Verification items for the finished model (mm, model axes). Round coordinates to 2 decimals unless told otherwise and drop trailing zeros. Loops run counter-clockwise (first coordinate to the right, second up) from the corner with the lowest first, then second, coordinate; pieces in that order, holes last. Notation, with made-up numbers: (-39.75, 39) - (-25.75, 39) arc R34 ccw to (-25.75, 69) - close; hole circle Ø8 at (49.5, 82). An arc over 180 degrees is marked (long way). Use a Markdown table: item, result. Add a question column.
```python
from build123d import *

# Parameters (mm, degrees)
F0_R      = 12
F1_DEPTH  = 2
F3_DEPTH  = 2
F4_R      = 1.5
F5_DEPTH  = 25
F6_R      = 6.35
F7_DEPTH  = 25
F8_R      = 1.5
F9_DEPTH  = 25
F10_R     = 1.5
F11_DEPTH = 25
F12_SIZE  = 1.86


with BuildPart() as f1:
    # F0 (on Front) → F1 (new body)
    with BuildSketch(Plane.XZ):
        with BuildLine():
            ThreePointArc((64.5, -22.5), (87, 0), (64.5, 22.5))
            Line((64.5, 22.5), (-64.5, 22.5))
            ThreePointArc((-64.5, 22.5), (-87, 0), (-64.5, -22.5))
            Line((-64.5, -22.5), (64.5, -22.5))
        make_face()
        with Locations((-64.5, 0)):
            Circle(F0_R, mode=Mode.SUBTRACT)
        with Locations((64.5, 0)):
            Circle(F0_R, mode=Mode.SUBTRACT)
    extrude(amount=F1_DEPTH)

    # F2 (on face) → F3 (join)
    with BuildSketch(Plane.XZ.offset(2)):
        Polygon((-87, -22.5), (-64.5, -22.5), (-64.5, -17.4313578755), (-70.5482587218, -14.7617282346), (-78.2682448626, -9.4630774111), (-80.8771923184, 0), (-87, 0), align=None)
    extrude(amount=-F3_DEPTH)

    # F4 (on face) → F5 (cut)
    with BuildSketch(Plane.XZ.offset(2)):
        with Locations((-53.5, 16)):
            Circle(F4_R)
        with Locations((-53.5, -16)):
            Circle(F4_R)
        with Locations((53.5, 16)):
            Circle(F4_R)
        with Locations((53.5, -16)):
            Circle(F4_R)
    extrude(amount=-F5_DEPTH, mode=Mode.SUBTRACT)

    # F6 (on face) → F7 (cut)
    with BuildSketch(Plane.XZ.offset(2)):
        Circle(F6_R)
    extrude(amount=-F7_DEPTH, mode=Mode.SUBTRACT)

    # F8 (on face) → F9 (cut)
    with BuildSketch(Plane.XZ.offset(2)):
        with Locations((-11.35, 4)):
            Circle(F8_R)
        with Locations((-11.35, -4)):
            Circle(F8_R)
        with Locations((11.35, 4)):
            Circle(F8_R)
        with Locations((11.35, -4)):
            Circle(F8_R)
    extrude(amount=-F9_DEPTH, mode=Mode.SUBTRACT)

    # F10 (on face) → F11 (cut)
    with BuildSketch(Plane.XZ.offset(2)):
        with Locations((0, -12.5)):
            Circle(F10_R)
        with Locations((31.499365073, -12.7)):
            Circle(F10_R)
        with Locations((-31.5, -12.5)):
            Circle(F10_R)
        with Locations((-37.5, -3.5)):
            Circle(F10_R)
    extrude(amount=-F11_DEPTH, mode=Mode.SUBTRACT)

    # F12
    f12_edges = [f1.edges().sort_by_distance(p)[0] for p in [
        (-55, 0, -16),
        (-33, 0, -12.5),
        (-55, 0, 16),
        (-12.85, 0, -4),
        (-12.85, 0, 4),
        (-1.5, 0, -12.5),
        (9.85, 0, -4),
        (9.85, 0, 4),
        (29.999365, 0, -12.7),
        (52, 0, -16),
        (52, 0, 16),
        (-39, 0, -3.5),
    ]]
    chamfer(f12_edges, length=F12_SIZE)


solid = f1.part
```
Q1. Thickness scan on line 1 along Z through (x, y) = (11.35, -1.85); line 2 along Z through (x, y) = (0, -1.85); line 3 along Z through (x, y) = (-64.5, -0.45). Record the ranges inside material, lowest first.
Q2. Release check for a two-part mould opening along Z. For faces 1 (the face through (-80.234, -0.986, 16.084)), 2 (the face through (-76.49, -0.99, 0.53)), 3 (the face through (-1, 0, 10)), 4 (the face through (87, -1, 0)) record: +Z half, -Z half, draft (parallel to the pull), parting line (faces both ways), or undercut.
Q3. Go/stop test with flat-tipped pins: pin 1 Ø3.5 at (x, z) = (-11.35, 4) entering from -Y; pin 2 Ø2.5 at (x, z) = (31.5, -12.7) entering from -Y; pin 3 Ø5 at (x, z) = (53.5, -16) entering from +Y; pin 4 Ø1 at (y, z) = (-1.5, 15) entering from -X. Record where each tip stops, or that it passes through.
Q4. Section check C-C on x = -63. Record the cut outline in (y, z).
Q5. Section check B-B on y = -0.7. State how many separate pieces and enclosed holes the cut face has, plus the area to 3 significant figures.
Q6. Section check A-A on x = 11.35. Record the cut outline in (y, z), plus the area to 3 significant figures.
Determined:
| question | item | result |
|---|---|---|
| 1 | line 1 | z = -22.5 to -5.51, -2.49 to 2.49, 5.51 to 22.5 |
| 1 | line 2 | z = -22.5 to -14.01, -10.99 to -6.35, 6.35 to 22.5 |
| 1 | line 3 | z = -22.5 to -12, 12 to 22.5 |
| 2 | face 1 | +Z half |
| 2 | face 2 | undercut |
| 2 | face 3 | draft |
| 2 | face 4 | parting line |
| 3 | pin 1 | stops at y = -2 |
| 3 | pin 2 | passes through |
| 3 | pin 3 | stops at y = -0.86 |
| 3 | pin 4 | stops at x = -81.7 |
| 4 | outline | (-2, -22.5) - (0, -22.5) - (0, -11.91) - (-2, -11.91) - close; (-2, 11.91) - (0, 11.91) - (0, 22.5) - (-2, 22.5) - close |
| 5 | separate pieces | 1 |
| 5 | enclosed holes | 15 |
| 5 | area | 6,210 mm² |
| 6 | outline | (-2, -22.5) - (0, -22.5) - (0, -7.36) - (-1.86, -5.5) - (-2, -5.5) - close; (-2, -2.5) - (-1.86, -2.5) - (0, -0.64) - (0, 0.64) - (-1.86, 2.5) - (-2, 2.5) - close; (-2, 5.5) - (-1.86, 5.5) - (0, 7.36) - (0, 22.5) - (-2, 22.5) - close |
| 6 | area | 71.1 mm² |
